Build history of the part. All positions in model axes, mm. A direction names the side the tool comes from. Coordinates: 2 decimals unless noted, no trailing zeros. Loops run counter-clockwise (first coordinate to the right, second up) from the corner with the lowest first, then second, coordinate; pieces in that order, holes last. Notation, with made-up numbers: (19, 80) -> (33, 80) arc R18 cw to (33, 112) -> close; hole circle Ø2 at (34, 61.25). An arc over 180 degrees is marked (long way). One line per item, written item: value. Start each with the question number.
```python
from build123d import *

# Parameters (mm, degrees)
SKETCH1_R                = 20
BOSS_EXTRUDE1_DEPTH      = 3.5
SKETCH2_R                = 35
SKETCH2_R_2              = 20
SKETCH2_R_3              = 2.8
BOSS_EXTRUDE2_DEPTH      = 8
BOSS_EXTRUDE3_DEPTH      = 2
BOSS_EXTRUDE3_DEPTH_BACK = 8
SKETCH4_R                = 2.9
SKETCH5_R                = 5
BOSS_EXTRUDE4_DEPTH      = 3
CUT_EXTRUDE1_START       = -10
SKETCH3_R                = 20
CUT_EXTRUDE1_DEPTH       = 10
SKETCH9_R                = 17.5
BOSS_EXTRUDE5_DEPTH      = 3.5
SKETCH10_R               = 17.5
SKETCH10_R_2             = 16.5
BOSS_EXTRUDE6_DEPTH      = 4.5
SKETCH11_W               = 2
SKETCH11_H               = 6.599117057
BOSS_EXTRUDE7_DEPTH      = 2
SKETCH12_R               = 72.135852014
CUT_EXTRUDE2_DEPTH       = 22
FILLET1_R                = 10


with BuildPart() as part:
    # Sketch1 → Boss-Extrude1 (new body)
    with BuildSketch(Plane(origin=(0, 0, 0), x_dir=(1, 0, 0), z_dir=(0, 1, 0))):
        with Locations(Location((0, 0, 0), (0, 0, 270))):
            Circle(SKETCH1_R)
    extrude(amount=BOSS_EXTRUDE1_DEPTH)

    # Sketch2 → Boss-Extrude2 (add)
    with BuildSketch(Plane(origin=(0, 0, 0), x_dir=(1, 0, 0), z_dir=(0, 1, 0))):
        with Locations(Location((0, 0, 0), (0, 0, 270))):
            Circle(SKETCH2_R)
        with Locations(Location((0, 0, 0), (0, 0, 270))):
            Circle(SKETCH2_R_2, mode=Mode.SUBTRACT)
        with Locations(Location((0, 29, 0), (0, 0, 270))):
            Circle(SKETCH2_R_3, mode=Mode.SUBTRACT)
        with Locations(Location((25.11473671, -14.5, 0), (0, 0, 270))):
            Circle(SKETCH2_R_3, mode=Mode.SUBTRACT)
        with Locations(Location((-25.11473671, -14.5, 0), (0, 0, 270))):
            Circle(SKETCH2_R_3, mode=Mode.SUBTRACT)
    extrude(amount=BOSS_EXTRUDE2_DEPTH)

    # Sketch4 → Boss-Extrude3 (add, two sides: drawn at the far end of the back side and taken through both)
    with BuildSketch(Plane.XZ.offset(-BOSS_EXTRUDE3_DEPTH_BACK)):
        with Locations(Location((-25.11473671, 14.5, 0), (0, 0, 270))):
            Circle(SKETCH4_R)
        with Locations(Location((25.11473671, 14.5, 0), (0, 0, 270))):
            Circle(SKETCH4_R)
        with Locations(Location((0, -29, 0), (0, 0, 270))):
            Circle(SKETCH4_R)
    extrude(amount=BOSS_EXTRUDE3_DEPTH + BOSS_EXTRUDE3_DEPTH_BACK)

    # Sketch5 → Boss-Extrude4 (add)
    with BuildSketch(Plane(origin=(0, 8, 0), x_dir=(1, 0, 0), z_dir=(0, 1, 0))):
        with Locations((-30.453629482, -17.250404383)):
            Circle(SKETCH5_R)
        with Locations((0.28752632, 34.99881896)):
            Circle(SKETCH5_R)
        with Locations((30.166103162, -17.748414577)):
            Circle(SKETCH5_R)
    extrude(amount=-BOSS_EXTRUDE4_DEPTH)

    # Sketch3 → Cut-Extrude1 (cut)
    with BuildSketch(Plane(origin=(0, 3.5, 0), x_dir=(1, 0, 0), z_dir=(0, 1, 0)).offset(CUT_EXTRUDE1_START)):
        with Locations(Location((0, 0, 0), (0, 0, 270))):
            Circle(SKETCH3_R)
    extrude(amount=CUT_EXTRUDE1_DEPTH, mode=Mode.SUBTRACT)



with BuildPart() as body_2:
    # Sketch9 → Boss-Extrude5 (new body)
    with BuildSketch(Plane(origin=(0, 8, 0), x_dir=(1, 0, 0), z_dir=(0, 1, 0))):
        with Locations(Location((0, 0, 0), (0, 0, 270))):
            Circle(SKETCH9_R)
    extrude(amount=-BOSS_EXTRUDE5_DEPTH)

    # Sketch10 → Boss-Extrude6 (add)
    with BuildSketch(Plane(origin=(0, 4.5, 0), x_dir=(-1, 0, 0), z_dir=(0, -1, 0))):
        with Locations(Location((0, 0, 0), (0, 0, 270))):
            Circle(SKETCH10_R)
        with Locations(Location((0, 0, 0), (0, 0, 270))):
            Circle(SKETCH10_R_2, mode=Mode.SUBTRACT)
    extrude(amount=BOSS_EXTRUDE6_DEPTH)


with BuildPart() as part_1:
    add(part.part)

    add(body_2.part)  # Boss-Extrude7 merges body 2
    # Sketch11 → Boss-Extrude7 (add)
    with BuildSketch(Plane(origin=(0, 8, 0), x_dir=(1, 0, 0), z_dir=(0, 1, 0))):
        Polygon((19.946286756, -10.36129349), (14.231283742, -7.061734961), (13.231283742, -8.793785769), (18.946286756, -12.093344297), align=None)
        with Locations((0, 19.155079259)):
            Rectangle(SKETCH11_W, SKETCH11_H)
        Polygon((-18.946286756, -12.093344297), (-13.231283742, -8.793785769), (-14.231283742, -7.061734961), (-19.946286756, -10.36129349), align=None)
    extrude(amount=-BOSS_EXTRUDE7_DEPTH)

    # Sketch12 → Cut-Extrude2 (cut)
    with BuildSketch(Plane(origin=(0, 8, 0), x_dir=(1, 0, 0), z_dir=(0, 1, 0))):
        Circle(SKETCH12_R)
        Polygon((0, 52), (-45.033320997, -26), (45.033320997, -26), align=None, mode=Mode.SUBTRACT)
    extrude(amount=-CUT_EXTRUDE2_DEPTH, mode=Mode.SUBTRACT)

    # Fillet1
    fillet1_edges = [part_1.edges().sort_by_distance(p)[0] for p in [
        (34.232035012, 4, 7.291623888),
        (10.801285985, 4, -33.291623888),
        (-23.430749028, 4, 26),
        (23.430749028, 4, 26),
        (-10.801285985, 4, -33.291623888),
        (-34.232035012, 4, 7.291623888),
    ]]
    fillet(fillet1_edges, radius=FILLET1_R)


solid = part_1.part
```
Item 1: Band-saw the part on B-B, the plane x = 0. List the corners of the cut face in (y, z).
Item 2: Band-saw the part on D-D, the plane x = 8. List the corners of the cut face in (y, z), and give its area (3 significant figures).
Item 3: Band-saw the part on A-A, the plane y = 2. List the corners of the cut face in (x, z), and give its area (3 significant figures).
Item 4: Two-plate mould, pull along Z, no slides. Class faces 4 (the face through (16, 6, 9)), 5 (the face through (0, 4, 26)), 6 (the face through (-16.7, 7.014, 8.487)), 7 (the face through (-32, 5, 18)): +Z half, -Z half, draft (parallel to the pull), parting line (faces both ways), or undercut.
Item 5: Band-saw the part on C-C, the plane z = 14.5. List the corners of the cut face in (x, y), and give its area (3 significant figures).
Item 6: Probe probe 1 along X at (y, z) = (7, 0.5); probe 2 along X at (y, z) = (5, -9); probe 3 along X at (y, z) = (1, -2.5). List the from-to ranges inside material, lowest first.
Item 7: Tool access for faces 1 (the face through (10.648, 4.056, -13.887)), 2 (the face through (9.922, 3.944, -32.873)), 3 (the face through (-1, 7, -19)): list every direction of +Z, -Z, +X, -X, +Y, -Y with a clear straight run to the whole face (end or side of a thin tool).
Item 8: Drop flat-ended pins along their axis: pin 1 Ø1.6 at (x, z) = (0.5, -37) entering from -Y; pin 2 Ø1.5 at (x, z) = (-15.5, 9) entering from -Y; pin 3 Ø2 at (y, z) = (5.5, -3.5) entering from +X. Give the stop position or say it passes through.
Worked out:
1. outline: (-2, -31.9) -> (0, -31.9) -> (0, -35) -> (5, -35) -> (5, -39.99) -> (8, -39.99) -> (8, 17.5) -> (0, 17.5) -> (0, 16.5) -> (4.5, 16.5) -> (4.5, -16.5) -> (0, -16.5) -> (0, -17.5) -> (6, -17.5) -> (6, -20) -> (0, -20) -> (0, -26.1) -> (-2, -26.1) -> close; (0, 20) -> (8, 20) -> (8, 26) -> (0, 26) -> close
2. outline: (0, -33.91) -> (8, -33.91) -> (8, -18.33) -> (0, -18.33) -> close; (0, -15.56) -> (8, -15.56) -> (8, 15.56) -> (0, 15.56) -> (0, 14.43) -> (4.5, 14.43) -> (4.5, -14.43) -> (0, -14.43) -> close; (0, 18.33) -> (8, 18.33) -> (8, 26) -> (0, 26) -> close
2. area: 305 mm²
3. outline: (-32.85, 12.09) arc R10 ccw to (-32.12, 3.64) -> (-12.91, -29.64) arc R10 ccw to (-5.95, -34.49) arc R35 ccw to (5.95, -34.49) arc R10 ccw to (12.91, -29.64) -> (32.12, 3.64) arc R10 ccw to (32.85, 12.09) arc R35 ccw to (26.89, 22.4) arc R10 ccw to (19.21, 26) -> (-19.21, 26) arc R10 ccw to (-26.89, 22.4) arc R35 ccw to start; circle Ø35 at (0, 0); hole circle Ø40 at (0, 0); hole circle Ø33 at (0, 0)
3. area: 1,820 mm²
4. face 4: undercut
4. face 5: +Z half
4. face 6: undercut
4. face 7: draft
5. outline: (-34.63, 5) -> (-31.86, 5) -> (-31.86, 0) -> (-28.01, 0) -> (-28.01, -2) -> (-22.21, -2) -> (-22.21, 0) -> (-13.77, 0) -> (-13.77, 8) -> (-34.63, 8) -> close; (-9.8, 0) -> (-7.87, 0) -> (-7.87, 4.5) -> (7.87, 4.5) -> (7.87, 0) -> (9.8, 0) -> (9.8, 8) -> (-9.8, 8) -> close; (13.77, 0) -> (22.21, 0) -> (22.21, -2) -> (28.01, -2) -> (28.01, 0) -> (31.86, 0) -> (31.86, 5) -> (33.97, 5) -> (33.97, 8) -> (13.77, 8) -> close
5. area: 413 mm²
6. probe 1: x = -30.31 to -19.99, -17.49 to 17.49, 19.99 to 30.31
6. probe 2: x = -24.83 to -17.86, -15.01 to 15.01, 17.86 to 24.83
6. probe 3: x = -28.58 to -19.84, -17.32 to -16.31, 16.31 to 17.32, 19.84 to 28.58
7. face 1: -Y
7. face 2: -Z, +X, +Y, -Y
7. face 3: +Y, -Y
8. pin 1: stops at y = 5
8. pin 2: stops at y = 0
8. pin 3: stops at x = 28.58
